```python
from build123d import *

# Parameters (mm, degrees)
F2_DEPTH  = 5.5
F4_DEPTH  = 20
F5_SIZE   = 1
F7_DEPTH  = 25.2006128335
F9_DEPTH  = 23.3118180281
F12_DEPTH = 3.481088538
F15_DEPTH = 3.4810885381


with BuildPart() as f2:
    # F1 (on Top) → F2 (new body)
    with BuildSketch(Plane.XY):
        Polygon((-59.9452278197, 75.287711217), (-65.4452278197, 75.287711217), (-65.4452278197, 52.2770658135), (-87.1952278197, 52.2770658135), (-87.1952278197, 75.5888838416), (-92.6952278197, 75.5888838416), (-92.6952278197, 19.2692689693), (-87.1952278197, 19.2692689693), (-87.1952278197, 44.4698818028), (-65.4452278197, 44.4698818028), (-65.4452278197, -24.712288783), (-59.9452278197, -24.712288783), (-59.9452278197, 44.4698818028), (-38.1952278197, 44.4698818028), (-38.1952278197, 19.2692689693), (-32.6952278197, 19.2692689693), (-32.6952278197, 75.5888838416), (-38.1952278197, 75.5888838416), (-38.1952278197, 52.2770658135), (-59.9452278197, 52.2770658135), align=None)
    extrude(amount=F2_DEPTH)

    # F3 (on face) → F4 (join)
    with BuildSketch(Plane.XZ.offset(24.712288783)):
        Polygon((-64.2827278197, 0.000369343), (-61.1077278197, 0.000369343), (-59.5202278197, 2.75), (-61.1077278197, 5.499630657), (-64.2827278197, 5.499630657), (-65.8702278197, 2.75), align=None)
    extrude(amount=F4_DEPTH)

    # F5
    f5_edges = [f2.edges().sort_by_distance(p)[0] for p in [
        (-62.695228, -44.712289, 0.000369),
        (-60.313978, -44.712289, 1.375185),
        (-60.313978, -44.712289, 4.124815),
        (-62.695228, -44.712289, 5.499631),
        (-65.076478, -44.712289, 4.124815),
        (-65.076478, -44.712289, 1.375185),
    ]]
    chamfer(f5_edges, length=F5_SIZE)

    # F6 (on face) → F7 (cut, through all)
    with BuildSketch(Plane.XZ.offset(-19.2692689693)):
        Polygon((-38.1952278197, 5.5), (-38.1952278197, 0), (-32.6952278197, 5.5), align=None)
        Polygon((-92.6952278197, 5.5), (-92.6952278197, 0), (-87.1952278197, 5.5), align=None)
    extrude(amount=-F7_DEPTH, mode=Mode.SUBTRACT)

    # F8 (on face) → F9 (cut, through all)
    with BuildSketch(Plane(origin=(0, 75.5888838416, 0), x_dir=(-1, 0, 0), z_dir=(0, 1, 0))):
        Polygon((32.6952278197, 0), (38.1952278197, 5.5), (32.6952278197, 5.5), align=None)
        Polygon((87.1952278197, 0), (92.6952278197, 5.5), (87.1952278197, 5.5), align=None)
    extrude(amount=-F9_DEPTH, mode=Mode.SUBTRACT)

    # F11 (on 3pt) → F12 (cut, through all)
    with BuildSketch(Plane(origin=(1.6556105831, 1.166343485, 1.6556105831), x_dir=(-0.3152867036, 0.8950913859, -0.3152867036), z_dir=(0.6329251887, 0.4458827323, 0.6329251887))):
        Polygon((57.1011218912, 30.8971918968), (48.3789018654, 27.0081046003), (57.1011218912, 23.1190173037), align=None)
    extrude(amount=F12_DEPTH, mode=Mode.SUBTRACT)

    # F14 (on 3pt) → F15 (cut, through all)
    with BuildSketch(Plane(origin=(-24.583315709, -17.3184385322, 24.5833157086), x_dir=(-0.3152867036, 0.8950913859, 0.3152867036), z_dir=(0.6329251887, 0.4458827323, -0.6329251887))):
        Polygon((69.0301809517, -65.5454241745), (77.7524009774, -61.6563368779), (69.0301809516, -57.7672495814), align=None)
    extrude(amount=-F15_DEPTH, mode=Mode.SUBTRACT)


solid = f2.part
```
For this review, take the finished solid that the model builds, in its own axes (mm). A direction names the side the tool comes from. Round coordinates to 2 decimals unless told otherwise and drop trailing zeros. Order: outer loops, then holes, each group sorted by start corner. A loop starts at its lowest first (then second) coordinate and runs counter-clockwise, first axis right, second up.
Q1. Mouldability with a two-part tool opening along X and no side actions: class faces 1 (the flat face through (-32.695, 36, 3)), 2 (the flat face through (-63, -44.712, 3)), 3 (the flat face through (-59.945, 9, 3)) as pulls with the +X half, pulls with the -X half, needs draft (parallel to the pull), parting line crosses it, or undercut.
Findings below:
face 1: pulls with the +X half
face 2: needs draft
face 3: undercut
Q2. Wall thickness on line 1 (X direction, y = 55, z = 1.5); line 2 (X direction, y = 65, z = 4); line 3 (Y direction, x = -87, z = 4): over which ranges is each line inside the solid? List them lowest first.
Findings below:
line 1: x = -92.7 to -88.7, -65.45 to -59.95, -38.2 to -34.2
line 2: x = -92.7 to -91.2, -65.45 to -59.95, -38.2 to -36.7
line 3: y = 44.47 to 52.28
Q3. We need section C-C, the plane x = -71.5. Give the boundary of the cut face in (y, z), plus the area to 3 significant figures.
Findings below:
outline: (44.47, 0) - (52.28, 0) - (52.28, 5.5) - (44.47, 5.5) - close
area: 42.9 mm2
Q4. Insertion check: P1, Ø5, axis at x = -70, y = 6, coming from the +Z side; P2, Ø1.6, axis at x = -76, z = 2, coming from the +Y side; P3, Ø1.6, axis at x = -89, z = 2.5, coming from the -Y side; P4, Ø1.6, axis at x = -47.5, z = 1.5, coming from the -Y side. Each pin has a flat end and moves straight along its axis. Give the tip position at first contact, or say it passes through.
Findings below:
P1: passes through
P2: stops at y = 52.28
P3: stops at y = 19.27
P4: stops at y = 44.47
Q5. Machinability: for faces 4 (the flat face through (-60.3, -34.1, 4.1)), 5 (the flat face through (-60.3, -34.1, 1.4)), 6 (the flat face through (-89, 19.269, 1)), 7 (the flat face through (-65.445, 64, 3)), which of the approach directions +Z, -Z, +X, -X, +Y, -Y give a long, thin tool a straight path to every point of the face, cutting with its end or side? Answer none if there is none.
Findings below:
face 4: +Z, +X, -Y
face 5: -Z, +X, -Y
face 6: +Z, -Z, -X, -Y
face 7: +Z, -Z, +Y
Q6. We need section A-A, the plane y = 58.5. Give the boundary of the cut face in (x, z), plus the area to 3 significant figures.
Findings below:
outline: (-92.7, 0) - (-87.2, 0) - (-92.7, 5.5) - close; (-65.45, 0) - (-59.95, 0) - (-59.95, 5.5) - (-65.45, 5.5) - close; (-38.2, 0) - (-32.7, 0) - (-38.2, 5.5) - close
area: 60.5 mm2
Q7. We need section B-B, the plane y = -26.5. Give the boundary of the cut face in (x, z), plus the area to 3 significant figures.
Findings below:
outline: (-65.87, 2.75) - (-64.28, 0) - (-61.11, 0) - (-59.52, 2.75) - (-61.11, 5.5) - (-64.28, 5.5) - close
area: 26.2 mm2
